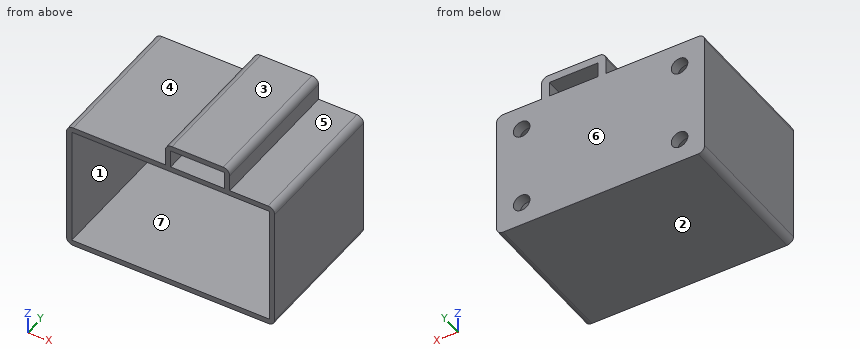
```python
from build123d import *

# Parameters (mm, degrees)
F0_W      = 78.5
F0_H      = 49
F0_W_2    = 74.5
F0_H_2    = 45
F1_DEPTH  = 53.7
F2_W      = 24.3
F2_H      = 10.7
F2_W_2    = 20.3
F2_H_2    = 6.7
F3_DEPTH  = 11.15
F5_DEPTH  = 1
F6_W      = 74.5
F6_H      = 45
F6_R      = 3.125
F7_DEPTH  = 4
F10_DEPTH = 42.55
F11_R     = 2.5


with BuildPart() as f1:
    # F0 (on Front) → F1 (new body)
    with BuildSketch(Plane.XZ):
        Rectangle(F0_W, F0_H)
        Rectangle(F0_W_2, F0_H_2, mode=Mode.SUBTRACT)
    extrude(amount=-F1_DEPTH)

    # F2 (on Front) → F3 (join)
    with BuildSketch(Plane.XZ):
        with Locations((10.15, 27.85)):
            Rectangle(F2_W, F2_H)
        with Locations((10.15, 27.85)):
            Rectangle(F2_W_2, F2_H_2, mode=Mode.SUBTRACT)
    extrude(amount=-F3_DEPTH)

    # F4 (on face) → F5 (join)
    with BuildSketch(Plane(origin=(0, 11.15, 0), x_dir=(-1, 0, 0), z_dir=(0, 1, 0))):
        Polygon((-20.3, 24.5), (-19.3, 24.5), (-19.3, 30.2), (-1, 30.2), (-1, 24.5), (0, 24.5), (0, 31.2), (-20.3, 31.2), align=None)
    extrude(amount=-F5_DEPTH)


with BuildPart() as f7:
    # F6 (on face) → F7 (new body)
    with BuildSketch(Plane(origin=(0, 53.7, 0), x_dir=(-1, 0, 0), z_dir=(0, 1, 0))):
        Rectangle(F6_W, F6_H)
        with Locations((-29.765, -15.355)):
            Circle(F6_R, mode=Mode.SUBTRACT)
        with Locations((29.765, -15.355)):
            Circle(F6_R, mode=Mode.SUBTRACT)
        with Locations((-29.765, 15.355)):
            Circle(F6_R, mode=Mode.SUBTRACT)
        with Locations((29.765, 15.355)):
            Circle(F6_R, mode=Mode.SUBTRACT)
    extrude(amount=-F7_DEPTH)

    # F8: union F1
    add(f1.part)

    # F9 (on face) → F10 (join, through all)
    with BuildSketch(Plane(origin=(0, 11.15, 0), x_dir=(-1, 0, 0), z_dir=(0, 1, 0))):
        Polygon((-22.3, 24.5), (-19.3, 24.5), (-19.3, 30.2), (-1, 30.2), (-1, 24.5), (2, 24.5), (2, 33.2), (-22.3, 33.2), align=None)
    extrude(amount=F10_DEPTH)

    # F11
    f11_edges = [f7.edges().sort_by_distance(p)[0] for p in [
        (22.3, 26.85, 33.2),
        (-2, 26.85, 33.2),
        (39.25, 26.85, 24.5),
        (39.25, 26.85, -24.5),
        (-39.25, 26.85, 24.5),
        (-39.25, 26.85, -24.5),
    ]]
    fillet(f11_edges, radius=F11_R)


solid = f7.part
```
Check sheet for the modelled part. Datum: model origin and axes. Units: mm. Face numbers are marked on the shaded views. A direction names the side the tool comes from. Give positions to 0.01 mm unless a question says otherwise; leave off trailing zeros. Order: outer loops, then holes, each group sorted by start corner. A loop starts at its lowest first (then second) coordinate and runs counter-clockwise, first axis right, second up. Notation, with made-up numbers: M -35,13 L -3,13 A30 ccw -3,47 Z; hole C 55.25,18.25 d3. An arc over 180 degrees is marked long. Answer in a Markdown table with one row per item. Add a question column.
Q1. Release check for a two-part mould opening along Z. For the marked faces 1, 2 and 3 record: released by +Z, released by -Z, zero draft, split by the parting line, or undercut.
Q2. Thickness scan on L1, parallel to Z at x = 12, y = 44; L2, parallel to X at y = 46, z = 21; L3, parallel to X at y = 26.5, z = 27. Record the ranges inside material, lowest first.
Q3. Sectioned sample at A-A, the plane y = 5. Record the boundary of the cut face in (x, z).
Q4. Sectioned sample at B-B, the plane x = 16. Record the boundary of the cut face in (y, z), and give its area (3 significant figures).
Q5. Sectioned sample at D-D, the plane x = 31. Record the boundary of the cut face in (y, z), and give its area (3 significant figures).
Q6. Gauge pin test, flat ends, axial feed: pin 1 Ø5.5 at (x, z) = (10, 27.5) entering from -Y; pin 2 Ø1.7 at (y, z) = (24.5, 28) entering from +X; pin 3 Ø5 at (x, z) = (29.765, -15.355) entering from +Y; pin 4 Ø15 at (x, y) = (-16.5, 33.5) entering from +Z. Record the tip position at first contact, or that the pin passes through.
Q7. Sectioned sample at C-C, the plane z = -9. Record the boundary of the cut face in (x, y), and give its area (3 significant figures).
Q8. Access from +Z, -Z, +X, -X, +Y, -Y to the whole of each face (thin tool, end or side, straight path). Record for the marked faces 4, 5, 6 and 7.
Verdict:
| question | item | result |
|---|---|---|
| 1 | face 1 | undercut |
| 1 | face 2 | released by -Z |
| 1 | face 3 | released by +Z |
| 2 | L1 | -24.5 to -22.5, 22.5 to 24.5, 30.2 to 33.2 |
| 2 | L2 | -39.25 to -37.25, 37.25 to 39.25 |
| 2 | L3 | -2 to 1, 19.3 to 22.3 |
| 3 | outline | M -39.25,-22 A2.5 ccw -36.75,-24.5 L 36.75,-24.5 A2.5 ccw 39.25,-22 L 39.25,22 A2.5 ccw 36.75,24.5 L 22.3,24.5 L 22.3,30.7 A2.5 ccw 19.8,33.2 L 0.5,33.2 A2.5 ccw -2,30.7 L -2,24.5 L -36.75,24.5 A2.5 ccw -39.25,22 Z; hole M -37.25,-22.5 L 37.25,-22.5 L 37.25,22.5 L -37.25,22.5 Z; hole M 0,24.5 L 20.3,24.5 L 20.3,31.2 L 0,31.2 Z |
| 4 | outline | M 0,-24.5 L 53.7,-24.5 L 53.7,24.5 L 0,24.5 L 0,22.5 L 49.7,22.5 L 49.7,-22.5 L 0,-22.5 Z; M 0,31.2 L 10.15,31.2 L 10.15,30.2 L 53.7,30.2 L 53.7,33.2 L 0,33.2 Z |
| 4 | area | 546 mm² |
| 5 | outline | M 0,-24.5 L 53.7,-24.5 L 53.7,-18.23 L 49.7,-18.23 L 49.7,-22.5 L 0,-22.5 Z; M 0,22.5 L 49.7,22.5 L 49.7,18.23 L 53.7,18.23 L 53.7,24.5 L 0,24.5 Z; M 49.7,-12.48 L 53.7,-12.48 L 53.7,12.48 L 49.7,12.48 Z |
| 5 | area | 349 mm² |
| 6 | pin 1 | y = 10.15 |
| 6 | pin 2 | x = 22.3 |
| 6 | pin 3 | through |
| 6 | pin 4 | z = 24.5 |
| 7 | outline | M -39.25,0 L -37.25,0 L -37.25,49.7 L 37.25,49.7 L 37.25,0 L 39.25,0 L 39.25,53.7 L -39.25,53.7 Z |
| 7 | area | 513 mm² |
| 8 | face 4 | +Z, -X, +Y, -Y |
| 8 | face 5 | +Z, +X, +Y, -Y |
| 8 | face 6 | +Z, -Z, +X, -X, +Y |
| 8 | face 7 | -Y |
